Answer from the drawing. Dimensions are ordinates in mm from the lowest x, y and z of the part. Give positions to 0.01 mm unless a question says otherwise; leave off trailing zeros. Order: outer loops, then holes, each group sorted by start corner. A loop starts at its lowest first (then second) coordinate and runs counter-clockwise, first axis right, second up.
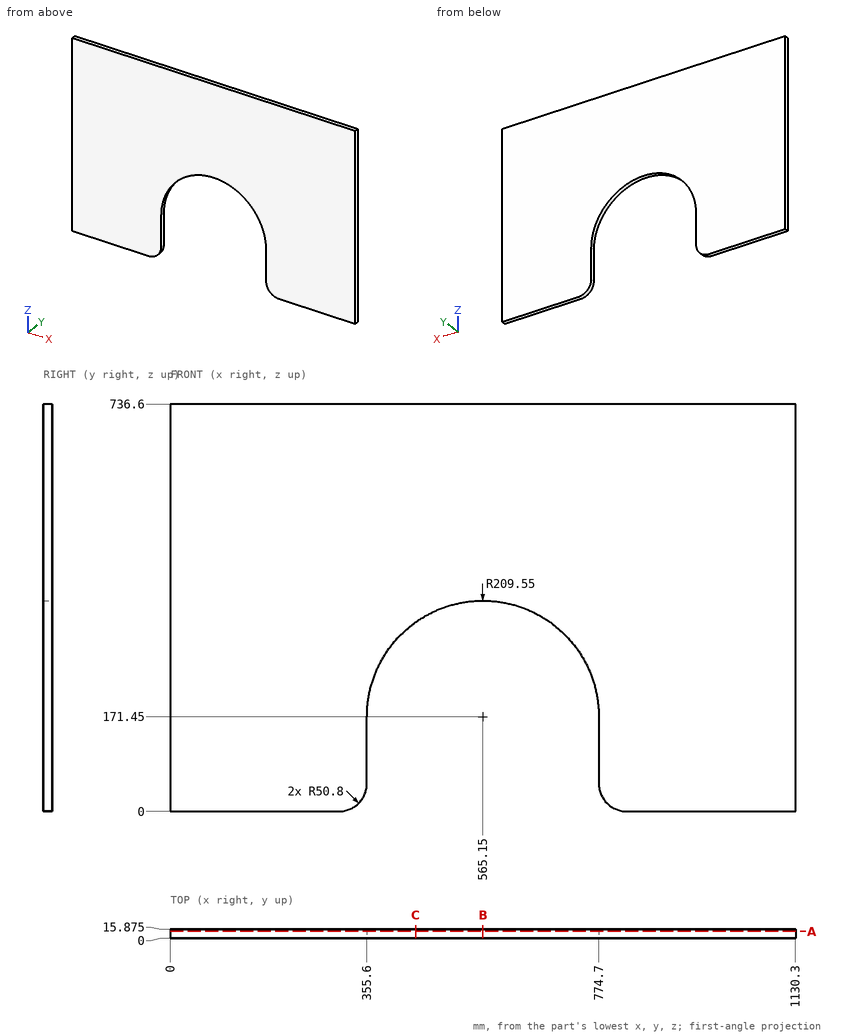
1) Consider L1, parallel to X at y = 11, z = 154.5; L2, parallel to X at y = 2.25, z = 220; L3, parallel to Z at x = 757.5, y = 10. Determine where each line is inside the solid, lowest interval first.
Final values:
L1: x = 0 to 355.6, 774.7 to 1130.3
L2: x = 0 to 361.3, 769 to 1130.3
L3: z = 254.59 to 736.6
2) Given pin 1 (3 mm diameter, centred on x = 328, y = 2.5, fed in from -Z); pin 2 (5 mm diameter, centred on x = 634, y = 4, fed in from -Z), each flat-ended and moving along its own axis, determine where each tip first touches the part or whether it passes through.
Final values:
pin 1: stops at z = 4.87
pin 2: stops at z = 368.48
3) The part is cut by section A-A on y = 12.5. Determine the outline of the cut face in (x, z).
Final values:
outline: (0, 0) - (304.8, 0) arc R50.8 ccw to (355.6, 50.8) - (355.6, 171.45) arc R209.55 cw to (774.7, 171.45) - (774.7, 50.8) arc R50.8 ccw to (825.5, 0) - (1130.3, 0) - (1130.3, 736.6) - (0, 736.6) - close
4) The part is cut by section C-C on x = 443.5. Determine the outline of the cut face in (y, z) (3 decimals).
Final values:
outline: (0, 342.074) - (15.875, 342.074) - (15.875, 736.6) - (0, 736.6) - close
5) The part is cut by section B-B on x = 565.15. Determine the outline of the cut face in (y, z) (3 decimals), and give its area (3 significant figures).
Final values:
outline: (0, 381) - (15.875, 381) - (15.875, 736.6) - (0, 736.6) - close
area: 5,650 mm2
